Read the model definition and answer for the solid it produces. Units are mm, in the model's axes. A direction names the side the tool comes from. Coordinates: 2 decimals unless noted, no trailing zeros. Order: outer loops, then holes, each group sorted by start corner. A loop starts at its lowest first (then second) coordinate and runs counter-clockwise, first axis right, second up. Notation, with made-up numbers: (-22, 3.5) - (-3, 3.5) arc R21 ccw to (-3, 7.5) - close; hole circle Ø11 at (40.25, 84). An arc over 180 degrees is marked (long way). Write item = value, one per line.
Autodesk Inventor part; units mm, degrees
ref_plane "YZ Plane" through (0, 0, 0) normal (1, 0, 0) x (0, 1, 0)
ref_plane "XZ Plane" through (0, 0, 0) normal (0, 1, 0) x (-1, 0, 0)
ref_plane "XY Plane" through (0, 0, 0) normal (0, 0, 1) x (1, 0, 0)
sketch "Sketch1" plane through (0, 0, 0) normal (0, 1, 0) x (-1, 0, 0)
  line L0 (-76.3737, 106.9555) -> (27.9763, 106.9555)
  line L1 (27.9763, 106.9555) -> (27.9763, -58.1445)
  line L2 (27.9763, -58.1445) -> (-76.3737, -58.1445)
  line L3 (-76.3737, -58.1445) -> (-76.3737, 106.9555)
  line L4 (-76.3737, 106.9555) -> (27.9763, -58.1445) construction
  line L5 (27.9763, 106.9555) -> (-76.3737, -58.1445) construction
  line L6 (38.2263, 114.9555) -> (38.2263, -66.9445)
  line L7 (38.2263, -66.9445) -> (-82.8737, -66.9445)
  line L8 (-82.8737, -66.9445) -> (-82.8737, 114.9555)
  line L9 (-82.8737, 114.9555) -> (38.2263, 114.9555)
  line L10 (41.2263, -69.9445) -> (41.2263, 117.9555)
  line L11 (41.2263, 117.9555) -> (-85.8737, 117.9555)
  line L12 (-85.8737, 117.9555) -> (-85.8737, -69.9445)
  line L13 (-85.8737, -69.9445) -> (41.2263, -69.9445)
  point P0 (-24.1987, 24.4055)
  dimension "d17" = 104.35
  dimension "d18" = 165.1
  dimension "d19" = 8.8
  dimension "d20" = 6.5
  dimension "d21" = 8
  dimension "d22" = 10.25
  dimension "d23" = 3
extrude "Extrusion1" add sketch "Sketch1" along normal blind 8.4 contours L6 L7 L8 L9 | L13 L12 L11 L10
extrude "Extrusion3" add sketch "Sketch1" against normal blind 10 contours L13 L12 L11 L10
fillet "Fillet3" radius 5 4 edges at (-41.2263, -0.8, 117.9555) (-41.2263, -0.8, -69.9445) (85.8737, -0.8, 117.9555) (85.8737, -0.8, -69.9445)
fillet "Fillet4" radius 3 8 edges at (22.3237, 8.4, -69.9445) (-39.7619, 8.4, -68.48) (-41.2263, 8.4, 24.0055) (-39.7619, 8.4, 116.491) (22.3237, 8.4, 117.9555) (84.4092, 8.4, 116.491) (85.8737, 8.4, 24.0055) (84.4092, 8.4, -68.48)
sketch "Sketch4" plane through (0, 0, 0) normal (0, -1, 0) x (1, 0, 0)
  line L0 (-38.2263, 112.9555) -> (-38.2263, -64.9445)
  line L1 (-27.9763, 106.9555) -> (-27.9763, -58.1445)
  line L2 (-38.2263, 64.9555) -> (-27.9763, 64.9555)
  line L3 (-27.9763, 64.9555) -> (-27.9763, 2.9555)
  line L4 (-27.9763, 2.9555) -> (-38.2263, 2.9555)
  line L5 (-38.2263, 2.9555) -> (-38.2263, 64.9555)
  line L6 (-38.2263, 114.9555) -> (82.8737, 114.9555)
  point P0 (0, 0)
  dimension "d28" = 50
  dimension "d29" = 62
extrude "Extrusion4" cut sketch "Sketch4" against normal blind 3.5
properties part number "top lcd mount"
1) The part is cut by section C-C (y = -3.25). Determine the outline of the cut face in (x, z).
Returned:
outline = (-41.23, -64.94) arc R5 ccw to (-36.23, -69.94) - (80.87, -69.94) arc R5 ccw to (85.87, -64.94) - (85.87, 112.96) arc R5 ccw to (80.87, 117.96) - (-36.23, 117.96) arc R5 ccw to (-41.23, 112.96) - close; hole (-38.23, -66.94) - (82.87, -66.94) - (82.87, 114.96) - (-38.23, 114.96) - close
2) Flat-ended cylindrical pins translate along their axes: pin 1 Ø3 at (x, z) = (-34.5, 37.5) entering from -Y; pin 2 Ø1 at (x, y) = (18, 6) entering from -Z. Find the tip coordinate at first contact, or state that the pin passes through.
Returned:
pin_1 = 3.5
pin_2 = -69.94
3) Straight lines are drawn through the part: line 1 along X through (y, z) = (-3.75, 101.5); line 2 along Z through (x, y) = (15, -7.5); line 3 along X through (y, z) = (2.25, 69). For each, find the intervals that lie inside material, in ascending order. Write a range as from..to.
Returned:
line_1 = -41.23..-38.23, 82.87..85.87
line_2 = -69.94..-66.94, 114.96..117.96
line_3 = -41.23..-27.98, 76.37..85.87
4) The part is cut by section D-D (x = -33). Determine the outline of the cut face in (y, z).
Returned:
outline = (-10, -69.94) - (5.4, -69.94) arc R3 ccw to (8.4, -66.94) - (8.4, 114.96) arc R3 ccw to (5.4, 117.96) - (-10, 117.96) - (-10, 114.96) - (0, 114.96) - (0, 64.96) - (3.5, 64.96) - (3.5, 2.96) - (0, 2.96) - (0, -66.94) - (-10, -66.94) - close
5) For faces 1 (the face through (81, 0, 24)), 2 (the face through (-39, -10, 24)), 3 (the face through (-27.976, 5, 26)), determine the directions among +Z, -Z, +X, -X, +Y, -Y from which every point of the face is accessible in a straight line to the end or side of a thin tool.
Returned:
face_1 = -Y
face_2 = +Z, -Z, +X, -X, -Y
face_3 = +Y, -Y
6) The part is cut by section B-B (z = 82.5). Determine the outline of the cut face in (x, y).
Returned:
outline = (-41.23, -10) - (-38.23, -10) - (-38.23, 0) - (-27.98, 0) - (-27.98, 8.4) - (-38.23, 8.4) arc R3 ccw to (-41.23, 5.4) - close; (76.37, 0) - (82.87, 0) - (82.87, -10) - (85.87, -10) - (85.87, 5.4) arc R3 ccw to (82.87, 8.4) - (76.37, 8.4) - close
7) The part is cut by section A-A (x = 43.5). Determine the outline of the cut face in (y, z).
Returned:
outline = (-10, -69.94) - (5.4, -69.94) arc R3 ccw to (8.4, -66.94) - (8.4, -58.14) - (0, -58.14) - (0, -66.94) - (-10, -66.94) - close; (-10, 114.96) - (0, 114.96) - (0, 106.96) - (8.4, 106.96) - (8.4, 114.96) arc R3 ccw to (5.4, 117.96) - (-10, 117.96) - close
8) Determine the mould class of faces 4 (the face through (84.37, -2.41, -68.52)), 5 (the face through (-41.226, -2, 23)), 6 (the face through (-38.226, -5, 25)) for opening direction Z: pulls with the +Z half, pulls with the -Z half, needs draft (parallel to the pull), parting line crosses it, or undercut.
Returned:
face_4 = pulls with the -Z half
face_5 = needs draft
face_6 = undercut
